```python
from build123d import *

# Parameters (mm, degrees)
CROQUIS1_W              = 44
CROQUIS1_H              = 25
SALIENTE_EXTRUIR2_DEPTH = 10
CROQUIS2_W              = 42
CROQUIS2_H              = 23
CORTAR_EXTRUIR1_DEPTH   = 9
CROQUIS3_W              = 1
CROQUIS3_H              = 2
SALIENTE_EXTRUIR3_DEPTH = 25
CROQUIS4_W              = 42
CROQUIS4_H              = 23
CORTAR_EXTRUIR2_DEPTH   = 28
CROQUIS5_W              = 1
CROQUIS5_H              = 23
CORTAR_EXTRUIR10_DEPTH  = 5
CROQUIS6_W              = 29.89343235
CROQUIS6_H              = 11.447342814
CORTAR_EXTRUIR11_DEPTH  = 1
CROQUIS7_W              = 31.003837105
CROQUIS7_H              = 9.868746677
CORTAR_EXTRUIR12_DEPTH  = 1
CROQUIS8_W              = 1
CROQUIS8_H              = 23
SALIENTE_EXTRUIR4_DEPTH = 5
CROQUIS9_W              = 8
CROQUIS9_H              = 4
CORTAR_EXTRUIR17_DEPTH  = 87


with BuildPart() as part:
    # Croquis1 → Saliente-Extruir2 (new body)
    with BuildSketch(Plane(origin=(0, 0, 0), x_dir=(1, 0, 0), z_dir=(0, 1, 0))):
        Rectangle(CROQUIS1_W, CROQUIS1_H)
    extrude(amount=SALIENTE_EXTRUIR2_DEPTH)

    # Croquis2 → Cortar-Extruir1 (cut)
    with BuildSketch(Plane(origin=(0, 10, 0), x_dir=(1, 0, 0), z_dir=(0, 1, 0))):
        Rectangle(CROQUIS2_W, CROQUIS2_H)
    extrude(amount=-CORTAR_EXTRUIR1_DEPTH, mode=Mode.SUBTRACT)

    # Croquis3 → Saliente-Extruir3 (add)
    with BuildSketch(Plane.XY.offset(12.5)):
        Polygon((-23, 10), (-22, 10), (-16, 10), (-20, 13.5), (-20, 15), (-23, 15), align=None)
        Polygon((20, 13.5), (16, 10), (22, 10), (23, 10), (23, 15), (20, 15), align=None)
        with Locations((-22.5, 9)):
            Rectangle(CROQUIS3_W, CROQUIS3_H)
        with Locations((22.5, 9)):
            Rectangle(CROQUIS3_W, CROQUIS3_H)
    extrude(amount=-SALIENTE_EXTRUIR3_DEPTH)

    # Croquis4 → Cortar-Extruir2 (cut)
    with BuildSketch(Plane(origin=(0, 1, 0), x_dir=(1, 0, 0), z_dir=(0, 1, 0))):
        Rectangle(CROQUIS4_W, CROQUIS4_H)
    extrude(amount=CORTAR_EXTRUIR2_DEPTH, mode=Mode.SUBTRACT)

    # Croquis5 → Cortar-Extruir10 (cut)
    with BuildSketch(Plane(origin=(0, 15, 0), x_dir=(1, 0, 0), z_dir=(0, 1, 0))):
        with Locations((-21.5, 0)):
            Rectangle(CROQUIS5_W, CROQUIS5_H)
        with Locations((21.5, 0)):
            Rectangle(CROQUIS5_W, CROQUIS5_H)
    extrude(amount=-CORTAR_EXTRUIR10_DEPTH, mode=Mode.SUBTRACT)

    # Croquis6 → Cortar-Extruir11 (cut)
    with BuildSketch(Plane(origin=(23, 0, 0), x_dir=(0, 0, -1), z_dir=(1, 0, 0))):
        with Locations((-0.524699003, 11.114026003)):
            Rectangle(CROQUIS6_W, CROQUIS6_H)
    extrude(amount=-CORTAR_EXTRUIR11_DEPTH, mode=Mode.SUBTRACT)

    # Croquis7 → Cortar-Extruir12 (cut)
    with BuildSketch(Plane.ZY.offset(23)):
        with Locations((-0.729719636, 12.255463236)):
            Rectangle(CROQUIS7_W, CROQUIS7_H)
    extrude(amount=-CORTAR_EXTRUIR12_DEPTH, mode=Mode.SUBTRACT)

    # Croquis8 → Saliente-Extruir4 (add)
    with BuildSketch(Plane(origin=(0, 10, 0), x_dir=(1, 0, 0), z_dir=(0, 1, 0))):
        with Locations((-21.5, 0)):
            Rectangle(CROQUIS8_W, CROQUIS8_H)
        with Locations((21.5, 0)):
            Rectangle(CROQUIS8_W, CROQUIS8_H)
    extrude(amount=SALIENTE_EXTRUIR4_DEPTH)

    # Croquis9 → Cortar-Extruir17 (cut)
    with BuildSketch(Plane.ZY.offset(22)):
        with Locations((0, 5)):
            Rectangle(CROQUIS9_W, CROQUIS9_H)
    extrude(amount=-CORTAR_EXTRUIR17_DEPTH, mode=Mode.SUBTRACT)


solid = part.part
```
Check sheet for the modelled part. Datum: model origin and axes. Units: mm. A direction names the side the tool comes from. Round coordinates to 2 decimals unless told otherwise and drop trailing zeros. Loops run counter-clockwise (first coordinate to the right, second up) from the corner with the lowest first, then second, coordinate; pieces in that order, holes last. Notation, with made-up numbers: (-17, -26) -> (20, -26) arc R24 ccw to (20, 8) -> close; hole circle Ø3 at (-31.5, 81). An arc over 180 degrees is marked (long way). Write item = value, one per line. Start each with the question number.
1) Thickness scan on probe 1 along X at (y, z) = (10.75, 1); probe 2 along Z at (x, y) = (13, 9); probe 3 along Y at (x, z) = (10.5, 8.25). Record the ranges inside material, lowest first.
2) Gauge pin test, flat ends, axial feed: pin 1 Ø3 at (y, z) = (3.5, 2) entering from +X; pin 2 Ø5 at (x, z) = (8, 6.5) entering from +Y; pin 3 Ø0.5 at (x, z) = (1, -12) entering from +Y. Record the tip position at first contact, or that the pin passes through.
3) Sectioned sample at C-C, the plane x = -5. Record the cut outline in (y, z), plus the area to 3 significant figures.
4) Sectioned sample at B-B, the plane y = 6. Record the cut outline in (x, z).
5) Sectioned sample at D-D, the plane y = 8.5. Record the cut outline in (x, z), plus the area to 3 significant figures.
6) Sectioned sample at A-A, the plane z = -2. Record the cut outline in (x, y), plus the area to 3 significant figures.
7) Set-up check for faces 4 (the flat face through (0, 6, 12.5)), 5 (the flat face through (-21.5, 5, -4)), 6 (the flat face through (18.028, 11.774, 12.007)), 7 (the flat face through (0, 7, 11.5)): record each of +Z, -Z, +X, -X, +Y, -Y from which the full face is reachable in a straight line by a thin tool's end or side.
8) Release check for a two-part mould opening along X. For faces 1 (the flat face through (-21.5, 15, -0.2)), 2 (the flat face through (-22, 7.4, 0.2)), 3 (the flat face through (-17.972, 11.726, -11.993)) record: released by +X, released by -X, zero draft, split by the parting line, or undercut.
Results are:
q1.probe_1 = -22 to -21, 21 to 22
q1.probe_2 = -12.5 to -11.5, 11.5 to 12.5
q1.probe_3 = 0 to 1
q2.pin_1 = 22
q2.pin_2 = 1
q2.pin_3 = 10
q3.outline = (0, -12.5) -> (10, -12.5) -> (10, -11.5) -> (1, -11.5) -> (1, 11.5) -> (10, 11.5) -> (10, 12.5) -> (0, 12.5) -> close
q3.area = 43.0 mm^2
q4.outline = (-22, -12.5) -> (22, -12.5) -> (22, -4) -> (21, -4) -> (21, -11.5) -> (-21, -11.5) -> (-21, -4) -> (-22, -4) -> close; (-22, 4) -> (-21, 4) -> (-21, 11.5) -> (21, 11.5) -> (21, 4) -> (22, 4) -> (22, 12.5) -> (-22, 12.5) -> close
q5.outline = (-22, -12.5) -> (22, -12.5) -> (22, 12.5) -> (-22, 12.5) -> close; hole (-21, -11.5) -> (21, -11.5) -> (21, 11.5) -> (-21, 11.5) -> close
q5.area = 134 mm^2
q6.outline = (-22, 0) -> (22, 0) -> (22, 3) -> (21, 3) -> (21, 1) -> (-21, 1) -> (-21, 3) -> (-22, 3) -> close; (-22, 7) -> (-21, 7) -> (-21, 15) -> (-22, 15) -> close; (21, 7) -> (22, 7) -> (22, 15) -> (21, 15) -> close
q6.area = 64.0 mm^2
q7.face_4 = +Z, +X, -X, +Y, -Y
q7.face_5 = +X, -X
q7.face_6 = +Z, -Z, +Y
q7.face_7 = +Y
q8.face_1 = zero draft
q8.face_2 = released by -X
q8.face_3 = undercut
